Part model, mm, in its own coordinate system. A direction names the side the tool comes from. Give positions to 0.01 mm unless a question says otherwise; leave off trailing zeros. Write each loop counter-clockwise with the first axis right and the second up, starting at its lowest first coordinate (ties: lowest second). Pieces come first, ordered by that corner, then holes. Notation, with made-up numbers: (-5, 55.5) - (18, 55.5) arc R8 cw to (18, 63.5) - close; hole circle Ø8 at (-3, 1). An arc over 180 degrees is marked (long way). Answer in a Markdown table with one row per item. Add a question column.
1. Probe line 1 along X through (y, z) = (1.3, -15); line 2 along X through (y, z) = (5.8, -25); line 3 along Z through (x, y) = (-75.5, 5.05). List the from-to ranges inside material, lowest first.
2. Which spindle directions (+Z, -Z, +X, -X, +Y, -Y) get a long thin tool onto all of the face, cutting with end or side? Do faces 1 (the flat face through (33, 3, -42)), 2 (the flat face through (24, 3, -90)), 3 (the flat face through (-33, 3, -54)). Say none if no direction does.
3. Band-saw the part on C-C on y = 2.75. State how many separate pieces and enclosed holes the cut face has, plus the area to 3 significant figures.
4. Band-saw the part on A-A on x = -95. Write the cut outline in (y, z).
5. Drop flat-ended pins along their axis: pin 1 Ø3 at (y, z) = (2, -93) entering from +X; pin 2 Ø1.8 at (y, z) = (3, -92) entering from -X; pin 3 Ø1.8 at (x, y) = (32, 3.5) entering from +Z. Give the stop position or say it passes through.
6. Band-saw the part on B-B on z = 15.5. Write the cut outline in (x, y), plus the area to 3 significant figures.
7. Band-saw the part on D-D on x = -24. Write the cut outline in (y, z), plus the area to 3 significant figures.
8. Pull direction X, two halves, no side cores. Call faces 4 (the flat face through (-30, 3, -69)), 5 (the flat face through (36, 3, 78)), 6 (the flat face through (-36, 3, -1)): released by +X, released by -X, zero draft, split by the parting line, or undercut.
Autodesk Inventor part; units mm, degrees
ref_plane "YZ Plane" through (0, 0, 0) normal (1, 0, 0) x (0, 1, 0)
ref_plane "XZ Plane" through (0, 0, 0) normal (0, 1, 0) x (-1, 0, 0)
ref_plane "XY Plane" through (0, 0, 0) normal (0, 0, 1) x (1, 0, 0)
sketch "Sketch1" plane through (0, 0, 0) normal (0, 1, 0) x (-1, 0, 0)
  line L0 (-30, 90) -> (30, 90)
  line L1 (30, 90) -> (30, -90)
  line L2 (30, -90) -> (-30, -90)
  line L3 (-30, -90) -> (-30, 90)
  line L4 (-30, 90) -> (30, -90) construction
  line L5 (30, 90) -> (-30, -90) construction
  line L6 (-30, 84) -> (-36, 84)
  line L7 (-36, 84) -> (-36, 72)
  line L8 (-36, 72) -> (-30, 72)
  line L9 (-30, 72) -> (-30, 84)
  line L10 (-36, 66) -> (-30, 66)
  line L11 (-30, 66) -> (-30, 54)
  line L12 (-30, 54) -> (-36, 54)
  line L13 (-36, 54) -> (-36, 66)
  line L14 (-30, 42) -> (-36, 42)
  line L15 (-36, 42) -> (-36, 30)
  line L16 (-36, 30) -> (-30, 30)
  line L17 (-30, 30) -> (-30, 42)
  line L18 (-30, 18) -> (-36, 18)
  line L19 (-36, 18) -> (-36, 6)
  line L20 (-36, 6) -> (-30, 6)
  line L21 (-30, 6) -> (-30, 18)
  line L22 (0, 0) -> (-5.6352, 0)
  line L23 (-5.6352, 0) -> (0, 0)
  line L24 (0, 0) -> (0, 8.7024)
  line L25 (-30, 90) -> (30, -90) construction
  line L26 (30, 84) -> (36, 84)
  line L27 (36, 84) -> (36, 72)
  line L28 (36, 72) -> (30, 72)
  line L29 (30, 72) -> (30, 84)
  line L30 (36, 66) -> (30, 66)
  line L31 (30, 66) -> (30, 54)
  line L32 (30, 54) -> (36, 54)
  line L33 (36, 54) -> (36, 66)
  line L34 (-30, -84) -> (-36, -84)
  line L35 (-36, -84) -> (-36, -72)
  line L36 (-36, -72) -> (-30, -72)
  line L37 (-30, -72) -> (-30, -84)
  line L38 (-36, -66) -> (-30, -66)
  line L39 (-30, -66) -> (-30, -54)
  line L40 (-30, -54) -> (-36, -54)
  line L41 (-36, -54) -> (-36, -66)
  line L42 (-30, -42) -> (-36, -42)
  line L43 (-36, -42) -> (-36, -30)
  line L44 (-36, -30) -> (-30, -30)
  line L45 (-30, -30) -> (-30, -42)
  line L46 (-30, -18) -> (-36, -18)
  line L47 (-36, -18) -> (-36, -6)
  line L48 (-36, -6) -> (-30, -6)
  line L49 (-30, -6) -> (-30, -18)
  line L50 (30, -84) -> (36, -84)
  line L51 (36, -84) -> (36, -72)
  line L52 (36, -72) -> (30, -72)
  line L53 (30, -72) -> (30, -84)
  line L54 (30, -54) -> (36, -54)
  line L55 (30, -66) -> (30, -54)
  line L56 (36, -66) -> (30, -66)
  line L57 (36, -54) -> (36, -66)
  line L58 (18, 90) -> (6, 90)
  line L59 (6, 90) -> (6, 96)
  line L60 (6, 96) -> (18, 96)
  line L61 (18, 96) -> (18, 90)
  line L62 (-18, 90) -> (-6, 90)
  line L63 (-6, 90) -> (-6, 96)
  line L64 (-6, 96) -> (-18, 96)
  line L65 (-18, 96) -> (-18, 90)
  line L66 (18, -90) -> (6, -90)
  line L67 (6, -90) -> (6, -96)
  line L68 (6, -96) -> (18, -96)
  line L69 (18, -96) -> (18, -90)
  line L70 (-18, -90) -> (-6, -90)
  line L71 (-6, -90) -> (-6, -96)
  line L72 (-6, -96) -> (-18, -96)
  line L73 (-18, -96) -> (-18, -90)
  line L74 (30, -48) -> (113, -48)
  line L75 (113, -48) -> (113, 48)
  line L76 (113, 48) -> (30, 48)
  line L77 (30, 48) -> (30, -48)
  line L78 (101, -36) -> (36, -36)
  line L79 (36, -36) -> (36, 36)
  line L80 (36, 36) -> (101, 36)
  line L81 (101, 36) -> (101, -36)
  circle A0 centre (32.55, 33) radius 1.15
  circle A1 centre (32.55, -33) radius 1.15
  point P0 (0, -8.7024)
  dimension "d0" = 60
  dimension "d1" = 180
  dimension "d2" = 6
  dimension "d3" = 6
  dimension "d4" = 12
  dimension "d5" = 12
  dimension "d6" = 12
  dimension "d7" = 12
  dimension "d8" = 12
  dimension "d9" = 6
  dimension "d10" = 12
  dimension "d17" = 6
  dimension "d19" = 6
  dimension "d20" = 6
  dimension "d21" = 6
  dimension "d22" = 12
  dimension "d23" = 12
  dimension "d24" = 12
  dimension "d25" = 6
  dimension "d26" = 65
  dimension "d27" = 12
  dimension "d28" = 2.3
  dimension "d29" = 3.45
  dimension "d30" = 3
extrude "Extrusion1" add sketch "Sketch1" along normal blind 6
equation "\"d22\" = d23"
equation "\"d24\" = d23"
properties part number "case_back" material "Acrylic, Clear"
Values:
| question | item | result |
|---|---|---|
| 1 | line 1 | x = -113 to -101, -36 to 36 |
| 1 | line 2 | x = -113 to -101, -36 to 30 |
| 1 | line 3 | z = -48 to -36, 36 to 48 |
| 2 | face 1 | +X, +Y, -Y |
| 2 | face 2 | -Z, +X, +Y, -Y |
| 2 | face 3 | -X, +Y, -Y |
| 3 | separate pieces | 1 |
| 3 | enclosed holes | 3 |
| 3 | area | 15,200 mm² |
| 4 | outline | (0, -48) - (6, -48) - (6, -36) - (0, -36) - close; (0, 36) - (6, 36) - (6, 48) - (0, 48) - close |
| 5 | pin 1 | stops at x = 18 |
| 5 | pin 2 | stops at x = -18 |
| 5 | pin 3 | stops at z = 84 |
| 6 | outline | (-113, 0) - (-101, 0) - (-101, 6) - (-113, 6) - close; (-36, 0) - (36, 0) - (36, 6) - (-36, 6) - close |
| 6 | area | 504 mm² |
| 7 | outline | (0, -90) - (6, -90) - (6, 90) - (0, 90) - close |
| 7 | area | 1,080 mm² |
| 8 | face 4 | released by -X |
| 8 | face 5 | released by +X |
| 8 | face 6 | undercut |
